Verification items for the finished model (mm, model axes). A direction names the side the tool comes from. Round coordinates to 2 decimals unless told otherwise and drop trailing zeros. Loops run counter-clockwise (first coordinate to the right, second up) from the corner with the lowest first, then second, coordinate; pieces in that order, holes last. Notation, with made-up numbers: M 58.25,-27 L 102.25,-27 A15 ccw 102.25,-1 Z; hole C 10,-15.5 d5. An arc over 180 degrees is marked long. One line per item, written item: value.
from build123d import *

# Parameters (mm, degrees)
SKETCH1_R                 = 6.35
BOSS_EXTRUDE1_DEPTH       = 6.95
SKETCH2_R                 = 7.542662581
SKETCH2_R_2               = 4
CUT_EXTRUDE1_DEPTH        = 1.35
SKETCH3_R                 = 7.419476018
SKETCH3_R_2               = 5.08
CUT_EXTRUDE2_DEPTH        = 1.8
F_2_0MM_DOWEL_HOLE1_D     = 2
F_2_0MM_DOWEL_HOLE1_DEPTH = 2
F_2_0MM_DOWEL_HOLE1_TIP   = 0.600860619


with BuildPart() as part:
    # Sketch1 → Boss-Extrude1 (new body)
    with BuildSketch(Plane(origin=(0, 0, 0), x_dir=(1, 0, 0), z_dir=(0, 1, 0))):
        with Locations(Location((0, 0, 0), (0, 0, 270))):
            Circle(SKETCH1_R)
    extrude(amount=BOSS_EXTRUDE1_DEPTH)

    # Sketch2 → Cut-Extrude1 (cut)
    with BuildSketch(Plane.XZ):
        Circle(SKETCH2_R)
        with Locations(Location((0, 0, 0), (0, 0, 270))):
            Circle(SKETCH2_R_2, mode=Mode.SUBTRACT)
    extrude(amount=-CUT_EXTRUDE1_DEPTH, mode=Mode.SUBTRACT)

    # Sketch3 → Cut-Extrude2 (cut)
    with BuildSketch(Plane(origin=(0, 6.95, 0), x_dir=(1, 0, 0), z_dir=(0, 1, 0))):
        Circle(SKETCH3_R)
        with Locations(Location((0, 0, 0), (0, 0, 270))):
            Circle(SKETCH3_R_2, mode=Mode.SUBTRACT)
    extrude(amount=-CUT_EXTRUDE2_DEPTH, mode=Mode.SUBTRACT)

    # Ø2.0mm Dowel Hole1
    with Locations(Plane(origin=(-1.779430565, 3.37, 6.09558257), x_dir=(0.95993426294, 0, 0.280225285859), z_dir=(-0.280225285859, 0, 0.95993426294))):
        with Locations((0, 0)):
            Hole(F_2_0MM_DOWEL_HOLE1_D / 2, depth=F_2_0MM_DOWEL_HOLE1_DEPTH)
            with Locations((0, 0, -(F_2_0MM_DOWEL_HOLE1_DEPTH + F_2_0MM_DOWEL_HOLE1_TIP / 2))):  # 118° drill point
                Cone(0, F_2_0MM_DOWEL_HOLE1_D / 2, F_2_0MM_DOWEL_HOLE1_TIP, mode=Mode.SUBTRACT)


solid = part.part
(1) Depth check by flat-ended pin: pin 1 Ø3 at (x, z) = (-5, 3) entering from -Y; pin 2 Ø4 at (y, z) = (4.5, -3.5) entering from +X; pin 3 Ø1 at (y, z) = (1, -5) entering from -X. Enter the tip coordinate at first touch or a pass-through.
Completed:
pin 1: stops at y = 1.35
pin 2: stops at x = 6.17
pin 3: stops at x = -4.33
(2) Sectioned sample at D-D on z = -4.25. Enter the section's corners in (x, y), and give its area (3 significant figures).
Completed:
outline: M -4.72,1.35 L 4.72,1.35 L 4.72,5.15 L 2.78,5.15 L 2.78,6.95 L -2.78,6.95 L -2.78,5.15 L -4.72,5.15 Z
area: 45.9 mm^2
(3) Sectioned sample at C-C on y = 6. Enter the section's corners in (x, z).
Completed:
outline: C 0,0 d10.16
(4) Sectioned sample at B-B on z = 0. Enter the section's corners in (x, y).
Completed:
outline: M -6.35,1.35 L -4,1.35 L -4,0 L 4,0 L 4,1.35 L 6.35,1.35 L 6.35,5.15 L 5.08,5.15 L 5.08,6.95 L -5.08,6.95 L -5.08,5.15 L -6.35,5.15 Z
(5) Tool access check on faces 1 (the face through (4.1, 1.35, -1.3)), 2 (the face through (0, 6.95, 0)). Record the directions out of +Z, -Z, +X, -X, +Y, -Y that give a thin tool (end or side, any length) a straight path to the whole face; none if there is none.
Completed:
face 1: -Y
face 2: +Z, -Z, +X, -X, +Y
(6) Sectioned sample at A-A on x = 0. Enter the section's corners in (y, z).
Completed:
outline: M 0,-4 L 1.35,-4 L 1.35,-6.35 L 5.15,-6.35 L 5.15,-5.08 L 6.95,-5.08 L 6.95,5.08 L 5.15,5.08 L 5.15,6.35 L 1.35,6.35 L 1.35,4 L 0,4 Z
(7) Thickness scan on L1, parallel to Y at x = 5, z = -1.25; L2, parallel to Y at x = 3, z = 2.75; L3, parallel to Y at x = -1, z = 3.75. Record the ranges inside material, lowest first. Write a range as from..to.
Completed:
L1: y = 1.35..5.15
L2: y = 1.35..6.95
L3: y = 0..3.17, 3.57..6.95
(8) Mould release check, pull along Y, two halves, no side actions. Record for faces 3 (the face through (-1.1, 3.54, 3.69)), 4 (the face through (2, 5.15, -5)), 5 (the face through (-1.939, 2.483, 4.994)), 6 (the face through (5.037, 6.063, -0.661)): +Y half, -Y half, draft (parallel to the pull), parting line (faces both ways), or undercut.
Completed:
face 3: undercut
face 4: +Y half
face 5: undercut
face 6: draft
